Here's how the part is built. I have some questions about the finished solid (model axes, mm). A direction names the side the tool comes from. Round coordinates to 2 decimals unless told otherwise and drop trailing zeros. Write each loop counter-clockwise with the first axis right and the second up, starting at its lowest first coordinate (ties: lowest second). Pieces come first, ordered by that corner, then holes. Notation, with made-up numbers: (6.5, -29.5) -> (17.5, -29.5) arc R23 ccw to (17.5, -4.5) -> close; hole circle Ø6 at (62, -10). An arc over 180 degrees is marked (long way). Answer as CSV lines item,"result".
from build123d import *

# Parameters (mm, degrees)
ESQUISSE1_W        = 10
ESQUISSE1_H        = 10
BOSS_EXTRU_1_DEPTH = 20
D_GAGEMENT_M3_51_D = 3.7
ESQUISSE2_W        = 10
ESQUISSE2_H        = 10
BOSS_EXTRU_2_DEPTH = 25
ESQUISSE4_R        = 4
BOSS_EXTRU_3_DEPTH = 9


with BuildPart() as part:
    # Esquisse1 → Boss.-Extru.1 (new body)
    with BuildSketch(Plane(origin=(0, 0, 0), x_dir=(1, 0, 0), z_dir=(0, 1, 0))):
        Rectangle(ESQUISSE1_W, ESQUISSE1_H)
    extrude(amount=BOSS_EXTRU_1_DEPTH)

    # Dégagement M3.51 (through all)
    with Locations(Plane(origin=(0, 0, -5), x_dir=(-1, 0, 0), z_dir=(0, 0, -1))):
        with Locations((0, 15), (0, 5)):
            Hole(D_GAGEMENT_M3_51_D / 2)

    # Esquisse2 → Boss.-Extru.2 (add)
    with BuildSketch(Plane.XZ):
        Rectangle(ESQUISSE2_W, ESQUISSE2_H)
    extrude(amount=BOSS_EXTRU_2_DEPTH)

    # Esquisse4 → Boss.-Extru.3 (add)
    with BuildSketch(Plane(origin=(0, -15, 5), x_dir=(1, 0, 0), z_dir=(0, 0, -1))):
        with Locations(Location((0, 1.5, 0), (0, 0, 180))):
            Circle(ESQUISSE4_R)
    extrude(amount=-BOSS_EXTRU_3_DEPTH)


solid = part.part
Item 1: For faces 1 (the flat face through (0, 20, 0)), 2 (the cylindrical face through (0.521, -12.534, 9.437)), which set-ups out of +Z, -Z, +X, -X, +Y, -Y let a thin tool reach every point of the face, with its end or its side?
Results found:
face 1,"+Z, -Z, +X, -X, +Y"
face 2,"+Z"
Item 2: Suppose I cut it at B-B, the plane y = 5. List the corners of the cut face in (x, z) for me.
Results found:
outline,"(-5, -5) -> (-1.85, -5) -> (-1.85, 5) -> (-5, 5) -> close; (1.85, -5) -> (5, -5) -> (5, 5) -> (1.85, 5) -> close"
Item 3: Will these pins go through, and if not, where does the flat tip stop? pin 1 (1.5 mm diameter, centred on x = 2, y = 15, fed in from +Z); pin 2 (5 mm diameter, centred on x = 0, z = 12, fed in from +Y); pin 3 (4.5 mm diameter, centred on x = 0, y = 15, fed in from -Z).
Results found:
pin 1,"stops at z = 5"
pin 2,"stops at y = -12.5"
pin 3,"stops at z = -5"
Item 4: If we mould it in two halves opening along X, with no side actions, what happens to faces 3 (the cylindrical face through (-0.241, 6.834, 0.07)), 4 (the cylindrical face through (-0.241, 16.834, 0.07)), 5 (the flat face through (-5, -2, 0)), 6 (the flat face through (5, -2, 0))? For each: pulls with the +X half, pulls with the -X half, needs draft (parallel to the pull), parting line crosses it, or undercut.
Results found:
face 3,"undercut"
face 4,"undercut"
face 5,"pulls with the -X half"
face 6,"pulls with the +X half"
Item 5: I need wall thicknesses on L1, parallel to Y at x = 0, z = 1.75; L2, parallel to Y at x = 1.25, z = -0.5; L3, parallel to Z at x = -1.5, y = -4. Which ranges of each line are inside material? Lowest first, please.
Results found:
L1,"y = -25 to 3.15, 6.85 to 13.15, 16.85 to 20"
L2,"y = -25 to 3.64, 6.36 to 13.64, 16.36 to 20"
L3,"z = -5 to 5"
Item 6: Suppose I cut it at C-C, the plane y = -16.5. List the corners of the cut face in (x, z) for me.
Results found:
outline,"(-5, -5) -> (5, -5) -> (5, 5) -> (4, 5) -> (4, 14) -> (-4, 14) -> (-4, 5) -> (-5, 5) -> close"
Item 7: Suppose I cut it at A-A, the plane x = 0. List the corners of the cut face in (y, z) for me, then the cut area to 3 significant figures.
Results found:
outline,"(-25, -5) -> (3.15, -5) -> (3.15, 5) -> (-12.5, 5) -> (-12.5, 14) -> (-20.5, 14) -> (-20.5, 5) -> (-25, 5) -> close; (6.85, -5) -> (13.15, -5) -> (13.15, 5) -> (6.85, 5) -> close; (16.85, -5) -> (20, -5) -> (20, 5) -> (16.85, 5) -> close"
area,"448 mm²"
Item 8: Suppose I cut it at D-D, the plane x = 2.75. List the corners of the cut face in (y, z) for me.
Results found:
outline,"(-25, -5) -> (20, -5) -> (20, 5) -> (-13.6, 5) -> (-13.6, 14) -> (-19.4, 14) -> (-19.4, 5) -> (-25, 5) -> close"
